from build123d import *
from build123d.topology import SkipClean

# Parameters (mm, degrees)
BOSS_EXTRUDE1_DEPTH = 93
SKETCH8_R           = 1.125
CUT_EXTRUDE1_DEPTH  = 124.766046621
CIRPATTERN1_COUNT   = 2
CIRPATTERN1_ANGLE   = 99
SKETCH9_R           = 1.125
CUT_EXTRUDE2_DEPTH  = 4
CUT_EXTRUDE3_START  = -5.2
CUT_EXTRUDE3_DEPTH  = 5.2
CUT_EXTRUDE4_START  = -0.1
CUT_EXTRUDE4_DEPTH  = 0.1
CUT_EXTRUDE5_DEPTH  = 0.1
CUT_EXTRUDE7_DEPTH  = 117.6697906


with BuildPart() as part:
    # Sketch1 → Boss-Extrude1 (new body)
    with BuildSketch(Plane(origin=(0, 0, 0), x_dir=(1, 0, 0), z_dir=(0, 1, 0))):
        with BuildLine():
            Line((43.301270189, 25), (42.262039705, 24.4))
            ThreePointArc((42.262039705, 24.4), (47.137180323, 12.630369401), (48.8, 0))
            ThreePointArc((48.8, 0), (47.137180323, -12.630369401), (42.262039705, -24.4))
            Line((42.262039705, -24.4), (43.301270189, -25))
            ThreePointArc((43.301270189, -25), (48.296291314, -12.940952255), (50, 0))
            ThreePointArc((50, 0), (48.296291314, 12.940952255), (43.301270189, 25))
        make_face()
        with BuildLine():
            ThreePointArc((0, 48.8), (24.4, 42.262039705), (42.262039705, 24.4))
            Line((42.262039705, 24.4), (43.301270189, 25))
            ThreePointArc((43.301270189, 25), (25, 43.301270189), (0, 50))
            Line((0, 50), (0, 48.8))
        make_face()
    extrude(amount=BOSS_EXTRUDE1_DEPTH)

    # Sketch8 → Cut-Extrude1 (cut, through all)
    with BuildSketch(Plane(origin=(47.132074555, 0, 16.690342962), x_dir=(0.33380685923377484, 0, -0.9426414910921771), z_dir=(0.9426414910921771, 0, 0.33380685923377484))):
        with Locations((0, 3)):
            Circle(SKETCH8_R)
    cut_extrude1 = extrude(amount=-CUT_EXTRUDE1_DEPTH, mode=Mode.SUBTRACT)

    # CirPattern1: Cut-Extrude1 ×2 about axis
    cirpattern1_axis = Axis((0, 93, 0), (0, 1, 0))
    for i in range(1, CIRPATTERN1_COUNT):
        add(cut_extrude1.rotate(cirpattern1_axis, i * CIRPATTERN1_ANGLE / (CIRPATTERN1_COUNT - 1)), mode=Mode.SUBTRACT)

    # Sketch9 → Cut-Extrude2 (cut)
    with SkipClean():  # the faces are left unmerged after this step: merging them gives an invalid solid
        with BuildSketch(Plane(origin=(43.301270189, 0, -25), x_dir=(-0.4999999999999981, 0, -0.8660254037844397), z_dir=(0.8660254037844398, 0, -0.4999999999999982))):
            with Locations((0, 90.5)):
                Circle(SKETCH9_R)
        extrude(amount=-CUT_EXTRUDE2_DEPTH, mode=Mode.SUBTRACT)

    # Sketch10 → Cut-Extrude3 (cut)
    with SkipClean():  # the faces are left unmerged after this step: merging them gives an invalid solid
        with BuildSketch(Plane(origin=(0, 93, 0), x_dir=(1, 0, 0), z_dir=(0, 1, 0)).offset(CUT_EXTRUDE3_START)):
            with BuildLine():
                ThreePointArc((45.681823724, -17.164235528), (44.120515076, -20.852341582), (42.262039705, -24.4))
                Line((42.262039705, -24.4), (43.301270189, -25))
                ThreePointArc((43.301270189, -25), (45.205445775, -21.365104079), (46.805147258, -17.586306893))
                Line((46.805147258, -17.586306893), (45.681823724, -17.164235528))
            make_face()
            with BuildLine():
                Line((0, 50), (0, 48.8))
                ThreePointArc((0, 48.8), (4.015214241, 48.634535616), (8.0032, 48.139264533))
                Line((8.0032, 48.139264533), (8.2, 49.323016939))
                ThreePointArc((8.2, 49.323016939), (4.113949017, 49.83046682), (0, 50))
            make_face()
        extrude(amount=CUT_EXTRUDE3_DEPTH, mode=Mode.SUBTRACT)

    # Sketch11 → Cut-Extrude4 (cut)
    with SkipClean():  # the faces are left unmerged after this step: merging them gives an invalid solid
        with BuildSketch(Plane(origin=(0, 93, 0), x_dir=(1, 0, 0), z_dir=(0, 1, 0)).offset(CUT_EXTRUDE4_START)):
            with BuildLine():
                Line((8.2, 49.323016939), (8.0032, 48.139264533))
                ThreePointArc((8.0032, 48.139264533), (42.26886825, 24.388168789), (45.681823724, -17.164235528))
                Line((45.681823724, -17.164235528), (46.805147258, -17.586306893))
                ThreePointArc((46.805147258, -17.586306893), (43.308266649, 24.987877858), (8.2, 49.323016939))
            make_face()
        extrude(amount=CUT_EXTRUDE4_DEPTH, mode=Mode.SUBTRACT)

    # Sketch1<3> → Cut-Extrude5 (cut)
    with SkipClean():  # the faces are left unmerged after this step: merging them gives an invalid solid
        with BuildSketch(Plane(origin=(0, 0, 0), x_dir=(1, 0, 0), z_dir=(0, 1, 0))):
            with BuildLine():
                Line((43.301270189, 25), (42.262039705, 24.4))
                ThreePointArc((42.262039705, 24.4), (47.137180323, 12.630369401), (48.8, 0))
                ThreePointArc((48.8, 0), (47.137180323, -12.630369401), (42.262039705, -24.4))
                Line((42.262039705, -24.4), (43.301270189, -25))
                ThreePointArc((43.301270189, -25), (48.296291314, -12.940952255), (50, 0))
                ThreePointArc((50, 0), (48.296291314, 12.940952255), (43.301270189, 25))
            make_face()
            with BuildLine():
                ThreePointArc((0, 48.8), (24.4, 42.262039705), (42.262039705, 24.4))
                Line((42.262039705, 24.4), (43.301270189, 25))
                ThreePointArc((43.301270189, 25), (25, 43.301270189), (0, 50))
                Line((0, 50), (0, 48.8))
            make_face()
        extrude(amount=CUT_EXTRUDE5_DEPTH, mode=Mode.SUBTRACT)

    # Sketch13 → Cut-Extrude7 (cut, through all)
    with SkipClean():  # the faces are left unmerged after this step: merging them gives an invalid solid
        with BuildSketch(Plane.XZ.offset(-0.1)):
            with BuildLine():
                Line((0.2, -49.999599998), (0.2, -48.799590162))
                ThreePointArc((0.2, -48.799590162), (0.10000021, -48.79989754), (0, -48.8))
                Line((0, -48.8), (0, -50))
                ThreePointArc((0, -50), (0.1000002, -49.9999), (0.2, -49.999599998))
            make_face()
            with BuildLine():
                Line((43.301270189, 25), (42.262039705, 24.4))
                ThreePointArc((42.262039705, 24.4), (42.311951077, 24.313346048), (42.361684775, 24.22659))
                Line((42.361684775, 24.22659), (43.400923778, 24.826594918))
                ThreePointArc((43.400923778, 24.826594918), (43.351183686, 24.913347286), (43.301270189, 25))
            make_face()
        extrude(amount=-CUT_EXTRUDE7_DEPTH, mode=Mode.SUBTRACT)


solid = part.part
Read the model definition and answer for the solid it produces. Units are mm, in the model's axes. Coordinates: 2 decimals unless noted, no trailing zeros. Write each loop counter-clockwise with the first axis right and the second up, starting at its lowest first coordinate (ties: lowest second). Pieces come first, ordered by that corner, then holes. Notation, with made-up numbers: M 49.25,89 L 105.25,89 A20 ccw 105.25,114 Z; hole C 89.25,87.5 d9. An arc over 180 degrees is marked long. Use a Markdown table: item, result.
Q1. Determine the mould class of faces 1 (the face through (46.93, 3.34, 15.48)), 2 (the face through (41.6, 0.1, -26.6)), 3 (the face through (42.9, 89.4, -24.5)), 4 (the face through (45, 87.8, 21)) for opening direction Y: released by +Y, released by -Y, zero draft, split by the parting line, or undercut.
Answer block:
| item | result |
|---|---|
| face 1 | undercut |
| face 2 | released by -Y |
| face 3 | undercut |
| face 4 | released by +Y |
Q2. The part is cut by section B-B, the plane z = -40. Write down the section's boundary in (x, y).
Answer block:
| item | result |
|---|---|
| outline | M 27.95,0.1 L 30,0.1 L 30,92.9 L 27.95,92.9 Z |
Q3. The part is cut by section A-A, the plane y = 14. Write down the section's boundary in (x, z), then the cut area to 3 significant figures.
Answer block:
| item | result |
|---|---|
| outline | M 0.2,-50 A50 ccw 43.4,24.83 L 42.36,24.23 A48.8 cw 0.2,-48.8 Z |
| area | 124 mm2 |
Q4. Straight lines are drawn through the part: L1, parallel to X at y = 65.5, z = 20.5; L2, parallel to Z at x = 22.5, y = 69; L3, parallel to X at y = 7.5, z = -38. For each, find the intervals that lie inside material, in ascending order. Write a range as [from, to].
Answer block:
| item | result |
|---|---|
| L1 | x = [44.29, 45.6] |
| L2 | z = [-44.65, -43.3] |
| L3 | x = [30.62, 32.5] |
Q5. Each of these flat-tipped pins is pushed along its axis until it touches: pin 1 Ø5 at (x, y) = (13.5, 19.5) entering from -Z (3 decimals); pin 2 Ø4 at (y, z) = (61.5, -20) entering from +X; pin 3 Ø4 at (y, z) = (71, -41) entering from -X. Where does it stop, or does it pass through?
Answer block:
| item | result |
|---|---|
| pin 1 | stops at z = -48.775 |
| pin 2 | stops at x = 46.65 |
| pin 3 | stops at x = 23.07 |
Q6. The part is cut by section C-C, the plane x = 17.5. Write down the section's boundary in (y, z), then the cut area to 3 significant figures.
Answer block:
| item | result |
|---|---|
| outline | M 0.1,-46.84 L 92.9,-46.84 L 92.9,-45.55 L 0.1,-45.55 Z |
| area | 119 mm2 |
